```python
from build123d import *

# Parameters (mm, degrees)
SKETCH1_R           = 2.75
BOSS_EXTRUDE1_DEPTH = 418
FILLET2_R           = 1
FILLET4_R           = 1
FILLET5_R           = 1
FILLET6_R           = 1


with BuildPart() as part:
    # Sketch1 → Boss-Extrude1 (new body)
    with BuildSketch(Plane.XY):
        Polygon((-3.001792446, 10), (-10, 10), (-10, 3.001792446), (-8.500771543, 3.001792446), (-8.500771543, 6.014407427), (-7.045753692, 6.014407427), (-4.458187435, 3.426841169), (-4.458187435, 0.939646666), (-3.934715846, 0), (-4.45749106, -0.939646666), (-4.458187435, -3.426841169), (-7.045753692, -6.014407427), (-8.500771543, -6.014407427), (-8.500771543, -3.001792446), (-10, -3.001792446), (-10, -10), (-3.001792446, -10), (-3.001792446, -8.499999951), (-6.014791508, -8.499999951), (-6.014791508, -7.045753643), (-3.427225251, -4.458187385), (-0.939604714, -4.458187385), (-0.00108721, -3.933944043), (0.937618184, -4.457850876), (3.425238721, -4.457850876), (6.012804978, -7.045417133), (6.012804978, -8.500000007), (3.001792545, -8.500000007), (3.001792545, -10), (16.998207455, -10), (16.998207455, -8.500000007), (13.987195022, -8.500000007), (13.987195022, -7.045417133), (16.574761279, -4.457850876), (19.062381816, -4.457850876), (20.00108721, -3.933944043), (20.939604714, -4.458187385), (23.427225251, -4.458187385), (26.014791508, -7.045753643), (26.014791508, -8.499999951), (23.001792446, -8.499999951), (23.001792446, -10), (30, -10), (30, -3.001792446), (28.500771543, -3.001792446), (28.500771543, -6.014407427), (27.045753692, -6.014407427), (24.458187435, -3.426841169), (24.45749106, -0.939646666), (23.934715846, 0), (24.458187435, 0.939646666), (24.458187435, 3.426841169), (27.045753692, 6.014407427), (28.500771543, 6.014407427), (28.500771543, 3.001792446), (30, 3.001792446), (30, 10), (23.001792446, 10), (23.001792446, 8.499999951), (26.014791508, 8.499999951), (26.014791508, 7.045753643), (23.427225251, 4.458187385), (20.939604714, 4.458187385), (20.00108721, 3.933944043), (19.062381816, 4.457850876), (16.574761279, 4.457850876), (13.987195022, 7.045417133), (13.987195022, 8.499999951), (16.998207356, 8.499999951), (16.998207356, 10), (3.001792643, 10), (3.001792643, 8.499999951), (6.012804978, 8.499999951), (6.012804978, 7.045417133), (3.425238721, 4.457850876), (0.937618184, 4.457850876), (-0.00108721, 3.933944043), (-0.939604714, 4.458187385), (-3.427225251, 4.458187385), (-6.014791508, 7.045753643), (-6.014791508, 8.499999951), (-3.001792446, 8.499999951), align=None)
        Circle(SKETCH1_R, mode=Mode.SUBTRACT)
        with Locations(Location((20, 0, 0), (0, 0, 180))):
            Circle(SKETCH1_R, mode=Mode.SUBTRACT)
        Polygon((7.208733292, -6.419793455), (7.208733292, -8.500000007), (12.791266708, -8.500000007), (12.791266708, -6.419793455), (15.541654987, -3.426231961), (15.541209058, -0.938611464), (16.065284154, 0), (15.54250894, 0.939646666), (15.541655044, 3.426231961), (12.791266708, 6.17760654), (12.791266708, 8.499999951), (7.208733292, 8.499999951), (7.208733292, 6.17760654), (4.458344956, 3.426231961), (4.45749106, 0.939646666), (3.934715846, 0), (4.458790942, -0.938611464), (4.458345013, -3.426231961), align=None, mode=Mode.SUBTRACT)
    extrude(amount=BOSS_EXTRUDE1_DEPTH)

    # Fillet2
    fillet2_edges = [part.edges().sort_by_distance(p)[0] for p in [
        (-10, -10, 209),
    ]]
    fillet(fillet2_edges, radius=FILLET2_R)

    # Fillet4
    fillet4_edges = [part.edges().sort_by_distance(p)[0] for p in [
        (-10, 10, 209),
    ]]
    fillet(fillet4_edges, radius=FILLET4_R)

    # Fillet5
    fillet5_edges = [part.edges().sort_by_distance(p)[0] for p in [
        (30, 10, 209),
    ]]
    fillet(fillet5_edges, radius=FILLET5_R)

    # Fillet6
    fillet6_edges = [part.edges().sort_by_distance(p)[0] for p in [
        (30, -10, 209),
    ]]
    fillet(fillet6_edges, radius=FILLET6_R)


solid = part.part
```
Here's how the part is built. I have some questions about the finished solid (model axes, mm). Coordinates: 2 decimals unless noted, no trailing zeros. One line per question, with ' | ' between items.
(1) If I drill on L1, parallel to X at y = -8.75, z = 123; L2, parallel to Y at x = 0, z = 150; L3, parallel to X at y = -6.25, z = 377.5, over which ranges is the centre line in solid material (lowest first)?
Report:
L1: x = -10 to -3, 3 to 17, 23 to 30 | L2: y = -3.93 to -2.75, 2.75 to 3.93 | L3: x = -10 to -5.22, 5.22 to 7.05, 12.95 to 14.78, 25.22 to 30
(2) If we mould it in two halves opening along Y, with no side actions, what happens to faces 1 (the flat face through (10, 10, 206)), 2 (the flat face through (10, -10, 206)), 3 (the flat face through (5, 5, 418))? For each: pulls with the +Y half, pulls with the -Y half, needs draft (parallel to the pull), parting line crosses it, or undercut.
Report:
face 1: pulls with the +Y half | face 2: pulls with the -Y half | face 3: needs draft
(3) Will this pin go through, and if not, where does the flat tip stop? pin 1 (1.5 mm diameter, centred on x = 18.5, z = 110, fed in from -Y).
Report:
pin 1: stops at y = -4.46
(4) Suppose I cut it at A-A on z = 268.5. State how many separate pieces and enclosed holes the cut face has, and give its area (3 significant figures).
Report:
separate pieces: 1 | enclosed holes: 3 | area: 294 mm2
